```python
from build123d import *

# Parameters (mm, degrees)
SKETCH1_R           = 7.5
BOSS_EXTRUDE1_DEPTH = 32.5
SKETCH4_R           = 12.5
BOSS_EXTRUDE3_DEPTH = 5


with BuildPart() as part:
    # Sketch1 → Boss-Extrude1 (new, symmetric)
    with BuildSketch(Plane(origin=(0, 0, 0), x_dir=(0, 0, -1), z_dir=(1, 0, 0))):
        Circle(SKETCH1_R)
    extrude(amount=BOSS_EXTRUDE1_DEPTH, both=True)

    # Sketch4 → Boss-Extrude3 (add)
    with BuildSketch(Plane(origin=(32.5, 0, 0), x_dir=(0, 0, -1), z_dir=(1, 0, 0))):
        Circle(SKETCH4_R)
    boss_extrude3 = extrude(amount=BOSS_EXTRUDE3_DEPTH)

    # Mirror1: Boss-Extrude3 across plane
    add(boss_extrude3.mirror(Plane(origin=(0, 0, 0), x_dir=(0, 0, 1), z_dir=(1, 0, 0))))


solid = part.part
```
The model under review builds one solid part; all positions refer to its coordinate system, in mm. A direction names the side the tool comes from. Round coordinates to 2 decimals unless told otherwise and drop trailing zeros. Loops run counter-clockwise (first coordinate to the right, second up) from the corner with the lowest first, then second, coordinate; pieces in that order, holes last. Notation, with made-up numbers: (8.25, 69) - (18.25, 69) arc R31 cw to (18.25, 98) - close; hole circle Ø7 at (30, -16.5). An arc over 180 degrees is marked (long way). Use a Markdown table: item, result. Add a question column.
Q1. The part is to be moulded in two halves that separate along X. For faces 3 (the face through (37.5, 0, 0)), 4 (the face through (-37.5, 0, 0)), 5 (the face through (-32.5, -8, 0)), 6 (the face through (34.965, 3.755, -11.923)), say which applies: pulls with the +X half, pulls with the -X half, needs draft (parallel to the pull), parting line crosses it, or undercut.
Q2. Add section B-B (z = 9.25). State the section outline as (x, y) points, plus the area to 3 significant figures.
Q3. Insertion check: pin 1 Ø4 at (x, y) = (26, 6.5) entering from +Z; pin 2 Ø5 at (x, y) = (-22.5, -6) entering from +Z; pin 3 Ø8 at (x, z) = (14.5, 1) entering from +Y. Each pin has a flat end and moves straight along its axis. Give the tip position at first contact, or say it passes through.
Q4. Add section A-A (y = 10). State the section outline as (x, z) points.
Q5. Add section C-C (z = 0). State the section outline as (x, y) points.
Q6. Machinability: for faces 1 (the face through (0.455, 0.33, 7.493)), 2 (the face through (-34.965, 3.755, -11.923)), which of the approach directions +Z, -Z, +X, -X, +Y, -Y give a long, thin tool a straight path to every point of the face, cutting with its end or side? Answer none if there is none.
Q7. For probe 1 along X at (y, z) = (-11, 2.5); probe 2 along Y at (x, z) = (-14.5, 0); probe 3 along Z at (x, y) = (-6, 4.25), list the stretches that pass through material, from the lowest coordinate up.
Worked answers:
| question | item | result |
|---|---|---|
| 1 | face 3 | pulls with the +X half |
| 1 | face 4 | pulls with the -X half |
| 1 | face 5 | undercut |
| 1 | face 6 | needs draft |
| 2 | outline | (-37.5, -8.41) - (-32.5, -8.41) - (-32.5, 8.41) - (-37.5, 8.41) - close; (32.5, -8.41) - (37.5, -8.41) - (37.5, 8.41) - (32.5, 8.41) - close |
| 2 | area | 168 mm² |
| 3 | pin 1 | z = 6 |
| 3 | pin 2 | z = 6.63 |
| 3 | pin 3 | y = 7.5 |
| 4 | outline | (-37.5, -7.5) - (-32.5, -7.5) - (-32.5, 7.5) - (-37.5, 7.5) - close; (32.5, -7.5) - (37.5, -7.5) - (37.5, 7.5) - (32.5, 7.5) - close |
| 5 | outline | (-37.5, -12.5) - (-32.5, -12.5) - (-32.5, -7.5) - (32.5, -7.5) - (32.5, -12.5) - (37.5, -12.5) - (37.5, 12.5) - (32.5, 12.5) - (32.5, 7.5) - (-32.5, 7.5) - (-32.5, 12.5) - (-37.5, 12.5) - close |
| 6 | face 1 | none |
| 6 | face 2 | +X, -X |
| 7 | probe 1 | -37.5 to -32.5, 32.5 to 37.5 |
| 7 | probe 2 | -7.5 to 7.5 |
| 7 | probe 3 | -6.18 to 6.18 |
